from build123d import *

# Parameters (mm, degrees)
BOSS_EXTRUDE1_DEPTH = 9.525
CUT_EXTRUDE1_REACH  = 337.179
SKETCH2_W           = 19.05
SKETCH2_H           = 6.35


with BuildPart() as part:
    # Sketch1 → Boss-Extrude1 (new, symmetric)
    with BuildSketch(Plane(origin=(0, 0, 0), x_dir=(1, 0, 0), z_dir=(0, 1, 0))):
        Polygon((-56.762661738, -101.318299445), (16.262338262, -101.318299445), (16.262338262, 228.881700555), (-5.962661738, 228.881700555), (-5.962661738, 178.081700555), (-56.762661738, 178.081700555), align=None)
    extrude(amount=BOSS_EXTRUDE1_DEPTH, both=True)

    # Sketch2 → Cut-Extrude1 (cut, up to next)
    with BuildSketch(Plane.XY.offset(101.318299445), mode=Mode.PRIVATE) as cut_extrude1_sk1:
        with Locations((6.737338262, 0)):
            Rectangle(SKETCH2_W, SKETCH2_H)
    cut_extrude1_tool1 = extrude(cut_extrude1_sk1.sketch, amount=-CUT_EXTRUDE1_REACH, mode=Mode.PRIVATE) & part.part
    add(cut_extrude1_tool1.solids().sort_by_distance((6.737338, 0, 101.318299))[0], mode=Mode.SUBTRACT)


solid = part.part
Can you work these out from the model? Positions are in its coordinate system, mm. A direction names the side the tool comes from. Coordinates: 2 decimals unless noted, no trailing zeros. Order: outer loops, then holes, each group sorted by start corner. A loop starts at its lowest first (then second) coordinate and runs counter-clockwise, first axis right, second up. Notation, with made-up numbers: M 4.25,31.5 L 40.25,31.5 A15 ccw 40.25,36.5 Z; hole C 54,72.25 d6. An arc over 180 degrees is marked long. Answer as CSV lines item,"result".
(1) I'm going to push flat-ended pins straight in: pin 1 (5.5 mm diameter, centred on x = -22, y = -2, fed in from -Z); pin 2 (5.5 mm diameter, centred on y = 2.5, z = -192, fed in from -X). Where does each tip first touch, or does it pass through?
Geometry check:
pin 1,"z = -178.08"
pin 2,"x = -5.96"
(2) Suppose I cut it at D-D on x = -13. Please give me the cut outline in (y, z) (3 decimals).
Geometry check:
outline,"M -9.525,-178.082 L 9.525,-178.082 L 9.525,101.318 L -9.525,101.318 Z"
(3) If we mould it in two halves opening along Y, with no side actions, what happens to faces 1 (the flat face through (16.262, -6, -61)), 2 (the flat face through (-2.788, 0, -61)), 3 (the flat face through (7, -3.175, -61)), 4 (the flat face through (-21, -9.525, -66))? For each: released by +Y, released by -Y, zero draft, split by the parting line, or undercut.
Geometry check:
face 1,"zero draft"
face 2,"undercut"
face 3,"undercut"
face 4,"released by -Y"
(4) Suppose I cut it at A-A on x = 3. Please give me the cut outline in (y, z) (3 decimals), plus the area to 3 significant figures.
Geometry check:
outline,"M -9.525,-228.882 L -3.175,-228.882 L -3.175,101.318 L -9.525,101.318 Z; M 3.175,-228.882 L 9.525,-228.882 L 9.525,101.318 L 3.175,101.318 Z"
area,"4,190 mm^2"
(5) On a 3-axis mill with a long thin cutter (end or side, diameter ignored), from which of +Z, -Z, +X, -X, +Y, -Y can I reach the whole of each face in a straight line? I mean faces 5 (the flat face through (-21, 0, 101.318)), 6 (the flat face through (-31, 0, -178.082)), 7 (the flat face through (7, 3.175, -61)). Say none if no direction works.
Geometry check:
face 5,"+Z, +X, -X, +Y, -Y"
face 6,"-Z, -X, +Y, -Y"
face 7,"+Z, -Z, +X"
(6) Suppose I cut it at C-C on y = -0.25. Please give me the cut outline in (x, z).
Geometry check:
outline,"M -56.76,-178.08 L -5.96,-178.08 L -5.96,-228.88 L -2.79,-228.88 L -2.79,101.32 L -56.76,101.32 Z"
(7) Suppose I cut it at B-B on z = -43. Please give me the cut outline in (x, y) (3 decimals).
Geometry check:
outline,"M -56.763,-9.525 L 16.262,-9.525 L 16.262,-3.175 L -2.788,-3.175 L -2.788,3.175 L 16.262,3.175 L 16.262,9.525 L -56.763,9.525 Z"
(8) Please list where these lines run through material, in increasing order: L1, parallel to Y at x = 4.5, z = -43 (3 decimals); L2, parallel to Z at x = -48, y = 4.75; L3, parallel to X at y = 0.25, z = 62.5.
Geometry check:
L1,"-9.525 to -3.175, 3.175 to 9.525"
L2,"-178.08 to 101.32"
L3,"-56.76 to -2.79"
